Geometry: final body of the model. Coordinates: model frame, mm. Round coordinates to 2 decimals unless told otherwise and drop trailing zeros. Loops run counter-clockwise (first coordinate to the right, second up) from the corner with the lowest first, then second, coordinate; pieces in that order, holes last. Notation, with made-up numbers: (23, -19.75) - (51, -19.75) arc R12 ccw to (51, -8.75) - close; hole circle Ø5 at (87.25, 36). An arc over 180 degrees is marked (long way). Return JSON: item names as keys, results as strings. Group by question number.
1. Material intervals for probe 1 along Y at (x, z) = (-6.4, 4); probe 2 along X at (y, z) = (-22, 3.25); probe 3 along Y at (x, z) = (-18.25, 3.25), sorted ascending.
2. Section C-C on z = 6.75. Return loops of the section in (x, y), and give its area (3 significant figures).
3. Section A-A on x = -20.4. Return loops of the section in (y, z).
4. First-contact query: pin 1 Ø4.5 at (x, y) = (-6.4, -20.4) entering from +Z. Flat tip, straight axial feed; report the tip coordinate or a pass-through.
5. Section B-B on y = -20.4. Return loops of the section in (x, z), and give its area (3 significant figures).
from build123d import *

# Parameters (mm, degrees)
F0_W     = 50.8
F0_H     = 50.8
F1_DEPTH = 13
F3_DEPTH = 16
F5_D     = 5


with BuildPart() as f1:
    # F0 (on Top) → F1 (new body)
    with BuildSketch(Plane.XY):
        Rectangle(F0_W, F0_H)
    extrude(amount=F1_DEPTH)

    # F2 (on face) → F3 (cut)
    with BuildSketch(Plane.XY.offset(13)):
        Polygon((-1.4, -5.4), (-1.4, -25.4), (25.4, -25.4), (25.4, 25.4), (-25.4, 25.4), (-25.4, -5.4), align=None)
    extrude(amount=-F3_DEPTH, mode=Mode.SUBTRACT)

    # F5 (through all)
    with Locations(Plane.XY.offset(13)):
        with Locations((-20.4, -10.4), (-20.4, -20.4), (-6.4, -10.4), (-6.4, -20.4)):
            Hole(F5_D / 2)


solid = f1.part
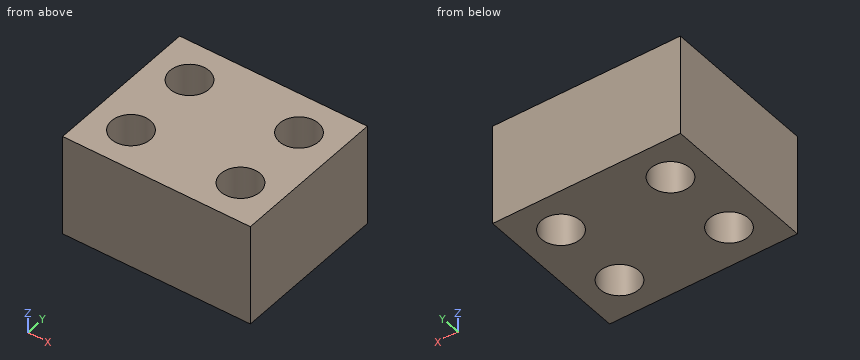
Taken from the geometry:
{
 "1": {"probe 1": "-25.4 to -22.9, -17.9 to -12.9, -7.9 to -5.4", "probe 2": "-25.4 to -22.32, -18.48 to -8.32, -4.48 to -1.4", "probe 3": "-25.4 to -21.68, -19.12 to -11.68, -9.12 to -5.4"},
 "2": {"outline": "(-25.4, -25.4) - (-1.4, -25.4) - (-1.4, -5.4) - (-25.4, -5.4) - close; hole circle Ø5 at (-20.4, -20.4); hole circle Ø5 at (-20.4, -10.4); hole circle Ø5 at (-6.4, -20.4); hole circle Ø5 at (-6.4, -10.4)", "area": "401 mm2"},
 "3": {"outline": "(-25.4, 0) - (-22.9, 0) - (-22.9, 13) - (-25.4, 13) - close; (-17.9, 0) - (-12.9, 0) - (-12.9, 13) - (-17.9, 13) - close; (-7.9, 0) - (-5.4, 0) - (-5.4, 13) - (-7.9, 13) - close"},
 "4": {"pin 1": "through"},
 "5": {"outline": "(-25.4, 0) - (-22.9, 0) - (-22.9, 13) - (-25.4, 13) - close; (-17.9, 0) - (-8.9, 0) - (-8.9, 13) - (-17.9, 13) - close; (-3.9, 0) - (-1.4, 0) - (-1.4, 13) - (-3.9, 13) - close", "area": "182 mm2"}
}
